Here's how the part is built. I have some questions about the finished solid (model axes, mm). Face numbers are marked on the shaded views. A direction names the side the tool comes from. Round coordinates to 2 decimals unless told otherwise and drop trailing zeros. Write each loop counter-clockwise with the first axis right and the second up, starting at its lowest first coordinate (ties: lowest second). Pieces come first, ordered by that corner, then holes. Notation, with made-up numbers: (-3, 35.5) - (20, 35.5) arc R33 ccw to (20, 74.5) - close; hole circle Ø3 at (44.5, -11). An arc over 180 degrees is marked (long way). Use one line per item in the form item = value. Start each with the question number.
1. If I drill on line 1 along X through (y, z) = (2.5, 17); line 2 along X through (y, z) = (23.5, 13); line 3 along Y through (x, z) = (44, 11), over which ranges is the centre line in solid material (lowest first)?
2. We'd pull the mould along X, two halves only. Please class the marked faces 4, 5 and 6: +X half, -X half, draft (parallel to the pull), parting line (faces both ways), or undercut.
3. I want a section at D-D, the plane z = 47.5. List the corners of the cut face in (x, y) for me, plus the area to 3 significant figures.
4. I want a section at C-C, the plane y = 0. List the corners of the cut face in (x, z) for me, plus the area to 3 significant figures.
5. I want a section at A-A, the plane z = 9.5. List the corners of the cut face in (x, y) for me.
6. Which directions (+Z, -Z, +X, -X, +Y, -Y) give clear straight access to the entire face, cutting with the end or side of a thin tool? Please do the marked faces 1, 2 and 3.
7. Will these pins go through, and if not, where does the flat tip stop? pin 1 (12.5 mm diameter, centred on x = 46, y = 8, fed in from +Z); pin 2 (2 mm diameter, centred on x = -8, y = -33, fed in from -Z); pin 3 (3 mm diameter, centred on x = -26.5, y = -32.5, fed in from +Z).
8. I want a section at B-B, the plane x = 22. List the corners of the cut face in (y, z) for me, plus the area to 3 significant figures.
```python
from build123d import *

# Parameters (mm, degrees)
F0_W      = 151.853732
F0_H      = 63.969113
F1_DEPTH  = 44.958
F2_T      = -5.08
F3_W      = 4.860878
F3_H      = 63.969113
F4_DEPTH  = 36.83
F5_R      = 28.577313
F6_DEPTH  = 2.54
F7_W      = 142.505951
F7_H      = 37.087826
F8_DEPTH  = 2.54
F9_W      = 3.11096
F9_H      = 53.809113
F10_DEPTH = 39.116


with BuildPart() as f1:
    # F0 (on Top) → F1 (new body)
    with BuildSketch(Plane.XY):
        with Locations((-0.097219, 0.583305)):
            Rectangle(F0_W, F0_H)
    extrude(amount=F1_DEPTH)

    # F2
    f2_openings = [f1.faces().sort_by_distance(p)[0] for p in [
        (-0.097219, 0.583306, 44.958),
    ]]
    offset(amount=F2_T, openings=f2_openings)

    # F3 (on face) → F4 (join)
    with BuildSketch(Plane.XY.offset(44.958)):
        with Locations((-73.593646, 0.583305)):
            Rectangle(F3_W, F3_H)
    extrude(amount=F4_DEPTH)

    # F5 (on face) → F6 (join)
    with BuildSketch(Plane(origin=(-76.024085, 0, 0), x_dir=(0, -1, 0), z_dir=(-1, 0, 0))):
        with Locations((0, 40.390089)):
            Circle(F5_R)
    extrude(amount=F6_DEPTH)

    # F7 (on face) → F8 (join)
    with BuildSketch(Plane.XZ.offset(31.401251)):
        with Locations((0.531253, 22.446518)):
            Rectangle(F7_W, F7_H)
    extrude(amount=F8_DEPTH)

    # F9 (on face) → F10 (join)
    with BuildSketch(Plane.XY.offset(5.08)):
        with Locations((26.816599, 0.583305)):
            Rectangle(F9_W, F9_H)
    extrude(amount=F10_DEPTH)


solid = f1.part
```
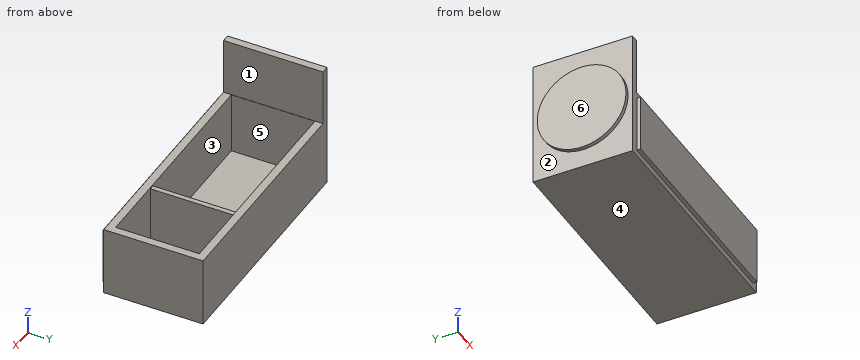
Model answer:
q1.line_1 = -78.56 to -70.94, 25.26 to 28.37, 70.75 to 75.83
q1.line_2 = -76.02 to -70.94, 25.26 to 28.37, 70.75 to 75.83
q1.line_3 = -33.94 to -26.32, 27.49 to 32.57
q2.face_4 = draft
q2.face_5 = undercut
q2.face_6 = -X half
q3.outline = (-78.56, -27.68) - (-76.02, -27.68) - (-76.02, -31.4) - (-71.16, -31.4) - (-71.16, 32.57) - (-76.02, 32.57) - (-76.02, 27.68) - (-78.56, 27.68) - close
q3.area = 452 mm2
q4.outline = (-78.56, 11.81) - (-76.02, 11.81) - (-76.02, 0) - (75.83, 0) - (75.83, 44.96) - (70.75, 44.96) - (70.75, 5.08) - (28.37, 5.08) - (28.37, 44.2) - (25.26, 44.2) - (25.26, 5.08) - (-70.94, 5.08) - (-70.94, 44.96) - (-71.16, 44.96) - (-71.16, 81.79) - (-76.02, 81.79) - (-76.02, 68.97) - (-78.56, 68.97) - close
q4.area = 1,620 mm2
q5.outline = (-76.02, -31.4) - (-70.72, -31.4) - (-70.72, -33.94) - (71.78, -33.94) - (71.78, -31.4) - (75.83, -31.4) - (75.83, 32.57) - (-76.02, 32.57) - close; hole (-70.94, -26.32) - (25.26, -26.32) - (25.26, 27.49) - (-70.94, 27.49) - close; hole (28.37, -26.32) - (70.75, -26.32) - (70.75, 27.49) - (28.37, 27.49) - close
q6.face_1 = +Z, +X, +Y, -Y
q6.face_2 = -X
q6.face_3 = +Z
q7.pin_1 = 5.08
q7.pin_2 = 3.9
q7.pin_3 = 44.96
q8.outline = (-33.94, 3.9) - (-31.4, 3.9) - (-31.4, 0) - (32.57, 0) - (32.57, 44.96) - (27.49, 44.96) - (27.49, 5.08) - (-26.32, 5.08) - (-26.32, 44.96) - (-31.4, 44.96) - (-31.4, 40.99) - (-33.94, 40.99) - close
q8.area = 824 mm2
